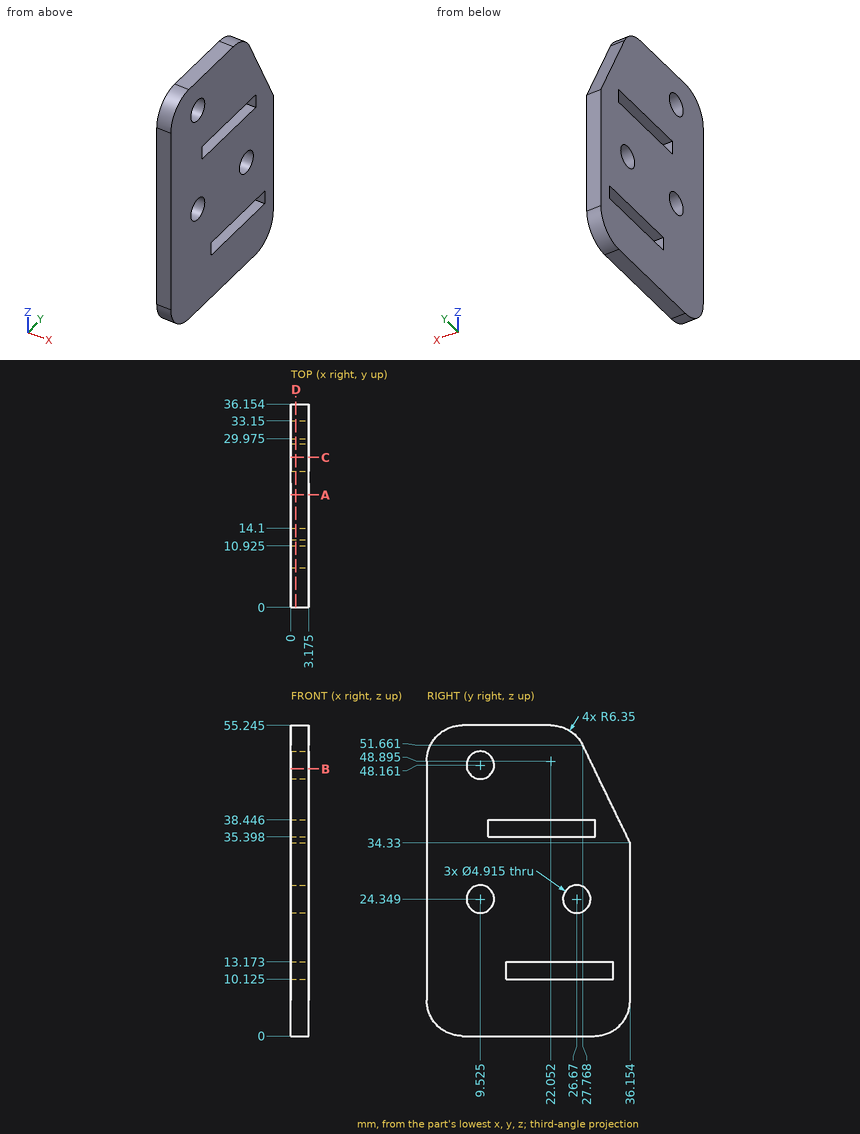
Study the drawing (mm; zero at the part's minimum x, y, z) and answer. Give positions to 0.01 mm unless a question says otherwise; leave off trailing zeros. Write each loop counter-clockwise with the first axis right and the second up, starting at its lowest first coordinate (ties: lowest second). Pieces come first, ordered by that corner, then holes. Notation, with made-up numbers: (70.5, 13) - (77.5, 13) arc R18 ccw to (77.5, 22) - close; hole circle Ø3 at (20, -7.5). An arc over 180 degrees is marked (long way). Use a Markdown table: item, result.
1. Section D-D on x = 0.9 is taken. Count the separate pieces of the cut face and the enclosed holes in it, plus the area to 3 significant figures.
Values follow:
| item | result |
|---|---|
| separate pieces | 1 |
| enclosed holes | 5 |
| area | 1,690 mm² |
2. Each of these flat-tipped pins is pushed along its axis until it touches: P1, Ø1, axis at x = 2, y = 24, coming from the -Z side; P2, Ø3, axis at y = 9.53, z = 48.16, coming from the +X side. Where does it stop, or does it pass through?
Values follow:
| item | result |
|---|---|
| P1 | stops at z = 0 |
| P2 | passes through |
3. Section C-C on y = 26.67 is taken. Write down the section's boundary in (x, z) (1 decimal).
Values follow:
| item | result |
|---|---|
| outline | (0, 0) - (3.2, 0) - (3.2, 10.1) - (0, 10.1) - close; (0, 13.2) - (3.2, 13.2) - (3.2, 21.9) - (0, 21.9) - close; (0, 26.8) - (3.2, 26.8) - (3.2, 35.4) - (0, 35.4) - close; (0, 38.4) - (3.2, 38.4) - (3.2, 53.3) - (0, 53.3) - close |
4. Section B-B on z = 47.5 is taken. Write down the section's boundary in (x, y) (1 decimal).
Values follow:
| item | result |
|---|---|
| outline | (0, 0) - (3.2, 0) - (3.2, 7.2) - (0, 7.2) - close; (0, 11.9) - (3.2, 11.9) - (3.2, 29.8) - (0, 29.8) - close |
5. Find the intervals of material crossed by probe 1 along Z at (x, y) = (2.2, 16.5) (1 decimal); probe 2 along Z at (x, y) = (0.85, 13.5) (1 decimal); probe 3 along Z at (x, y) = (3.05, 28) (1 decimal), in increasing order. Write a range as from..to.
Values follow:
| item | result |
|---|---|
| probe 1 | z = 0..10.1, 13.2..35.4, 38.4..55.2 |
| probe 2 | z = 0..35.4, 38.4..55.2 |
| probe 3 | z = 0..10.1, 13.2..22.3, 26.4..35.4, 38.4..51.2 |
6. Section A-A on y = 20 is taken. Write down the section's boundary in (x, z) (1 decimal).
Values follow:
| item | result |
|---|---|
| outline | (0, 0) - (3.2, 0) - (3.2, 10.1) - (0, 10.1) - close; (0, 13.2) - (3.2, 13.2) - (3.2, 35.4) - (0, 35.4) - close; (0, 38.4) - (3.2, 38.4) - (3.2, 55.2) - (0, 55.2) - close |
